The listing builds one solid part. Answer for the finished solid, in the listing's coordinates (mm). Coordinates: 2 decimals unless noted, no trailing zeros. Loops run counter-clockwise (first coordinate to the right, second up) from the corner with the lowest first, then second, coordinate; pieces in that order, holes last. Notation, with made-up numbers: M 83,71.25 L 126,71.25 A9 ccw 126,80.25 Z; hole C 6.5,62.5 d7. An arc over 180 degrees is marked long. Answer as a JSON object with one key per item and string values. Group by question number.
1. A cutting plane is placed at A-A on x = 1.55. Give the vertices of the cut face in (y, z).
2. Given pin 1 (1 mm diameter, centred on x = 1, z = -39.5, fed in from +Y), flat-ended and moving along its own axis, determine where the tip first touches the part or whether it passes through.
3. Straight lines are drawn through the part: L1, parallel to Z at x = 1.4, y = 3.5; L2, parallel to Y at x = 0.8, z = -121.5. For each, find the intervals that lie inside material, in ascending order.
4. A cutting plane is placed at B-B on z = 116. Give the vertices of the cut face in (x, y), and give its area (3 significant figures).
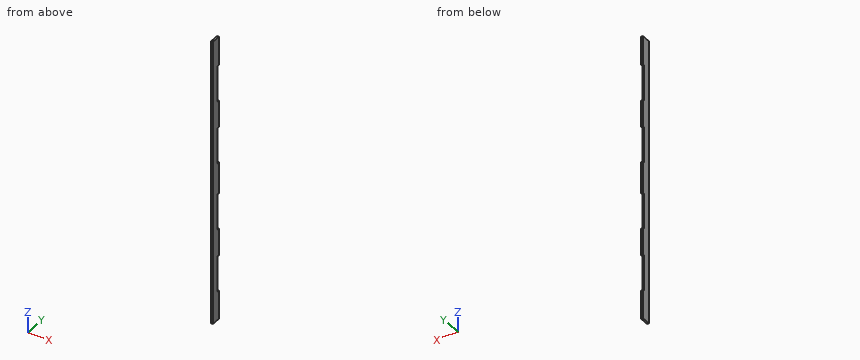
from build123d import *

# Parameters (mm, degrees)
SKETCH1_W               = 319
SKETCH1_H               = 10
BOSS_EXTRUDE1_DEPTH     = 2
CUT_EXTRUDE1_DEPTH      = 160.590883198
CUT_EXTRUDE1_DEPTH_BACK = 160.590883198
SKETCH2_W               = 40
SKETCH2_H               = 2


with BuildPart() as part:
    # Sketch1 → Boss-Extrude1 (new body)
    with BuildSketch(Plane(origin=(0, 0, 0), x_dir=(0, 0, -1), z_dir=(1, 0, 0))):
        Rectangle(SKETCH1_W, SKETCH1_H)
    extrude(amount=BOSS_EXTRUDE1_DEPTH)

    # Sketch2 → Cut-Extrude1 (cut, two sides: drawn at the far end of the back side and taken through both)
    with BuildSketch(Plane(origin=(2, 0, 0), x_dir=(0, 0, -1), z_dir=(1, 0, 0)).offset(-CUT_EXTRUDE1_DEPTH_BACK)):
        with Locations((-107.5, 4)):
            Rectangle(SKETCH2_W, SKETCH2_H)
        with Locations((-37.5, 4)):
            Rectangle(SKETCH2_W, SKETCH2_H)
        with Locations((37.5, 4)):
            Rectangle(SKETCH2_W, SKETCH2_H)
        with Locations((107.5, 4)):
            Rectangle(SKETCH2_W, SKETCH2_H)
    extrude(amount=CUT_EXTRUDE1_DEPTH + CUT_EXTRUDE1_DEPTH_BACK, mode=Mode.SUBTRACT)


solid = part.part
From the geometry:
{
 "1": {"outline": "M -5,-159.5 L 5,-159.5 L 5,-127.5 L 3,-127.5 L 3,-87.5 L 5,-87.5 L 5,-57.5 L 3,-57.5 L 3,-17.5 L 5,-17.5 L 5,17.5 L 3,17.5 L 3,57.5 L 5,57.5 L 5,87.5 L 3,87.5 L 3,127.5 L 5,127.5 L 5,159.5 L -5,159.5 Z"},
 "2": {"pin 1": "stops at y = 3"},
 "3": {"L1": "z = -159.5 to -127.5, -87.5 to -57.5, -17.5 to 17.5, 57.5 to 87.5, 127.5 to 159.5", "L2": "y = -5 to 3"},
 "4": {"outline": "M 0,-5 L 2,-5 L 2,3 L 0,3 Z", "area": "16.0 mm²"}
}
